from build123d import *

# Parameters (mm, degrees)
BOSS_EXTRUDE1_DEPTH = 5.9944
CUT_EXTRUDE2_DEPTH  = 5.9944


with BuildPart() as part:
    # Sketch1 → Boss-Extrude1 (new body)
    with BuildSketch(Plane.XY):
        Polygon((25.4, 5.9944), (50.8, 5.9944), (50.8, 0), (76.2, 0), (76.2, 5.9944), (101.6, 5.9944), (101.6, 0), (127, 0), (127, 75.4888), (101.6, 75.4888), (101.6, 69.4944), (76.2, 69.4944), (76.2, 75.4888), (50.8, 75.4888), (50.8, 69.4944), (25.4, 69.4944), (25.4, 75.4888), (0, 75.4888), (0, 0), (25.4, 0), align=None)
    extrude(amount=BOSS_EXTRUDE1_DEPTH)

    # Sketch2 → Cut-Extrude2 (cut)
    with BuildSketch(Plane.XY.offset(5.9944)):
        Polygon((36.449, 69.4944), (36.449, 64.4144), (34.163, 64.4144), (34.163, 61.8744), (36.449, 61.8744), (36.449, 58.0644), (39.751, 58.0644), (39.751, 61.8744), (42.037, 61.8744), (42.037, 64.4144), (39.751, 64.4144), (39.751, 69.4944), align=None)
        Polygon((36.449, 5.9944), (39.751, 5.9944), (39.751, 11.0744), (42.037, 11.0744), (42.037, 13.6144), (39.751, 13.6144), (39.751, 17.4244), (36.449, 17.4244), (36.449, 13.6144), (34.163, 13.6144), (34.163, 11.0744), (36.449, 11.0744), align=None)
        Polygon((90.551, 5.9944), (90.551, 11.0744), (92.837, 11.0744), (92.837, 13.6144), (90.551, 13.6144), (90.551, 17.4244), (87.249, 17.4244), (87.249, 13.6144), (84.963, 13.6144), (84.963, 11.0744), (87.249, 11.0744), (87.249, 5.9944), align=None)
        Polygon((90.551, 69.4944), (87.249, 69.4944), (87.249, 64.4144), (84.963, 64.4144), (84.963, 61.8744), (87.249, 61.8744), (87.249, 58.0644), (90.551, 58.0644), (90.551, 61.8744), (92.837, 61.8744), (92.837, 64.4144), (90.551, 64.4144), align=None)
    extrude(amount=-CUT_EXTRUDE2_DEPTH, mode=Mode.SUBTRACT)


solid = part.part
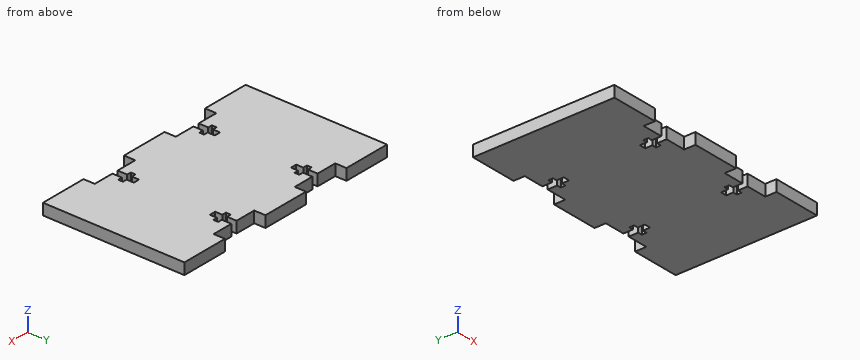
Input: part model. Units: mm. Frame: model coordinates. Coordinates: 2 decimals unless noted, no trailing zeros. Loops run counter-clockwise (first coordinate to the right, second up) from the corner with the lowest first, then second, coordinate; pieces in that order, holes last. Notation, with made-up numbers: (21.25, 50.25) - (67.25, 50.25) arc R31 ccw to (67.25, 80.25) - close; hole circle Ø2 at (1.25, 3.5). An arc over 180 degrees is marked (long way). Answer in a Markdown table with one row per item. Add a question column.
Item 1: Line query: line 1 along X through (y, z) = (70.5, 1.65); line 2 along X through (y, z) = (8.5, 3.8); line 3 along Y through (x, z) = (35.5, 0.8). Output: solid intervals per line, ascending. Write a range as [from, to].
Item 2: Contact query for flat-ended pins moving along their axis: P1, Ø1, axis at x = 15, y = 50, coming from the -Z side; P2, Ø1.1, axis at x = 86, z = 1.5, coming from the -Y side; P3, Ø0.7, axis at x = 91.5, z = 4, coming from the +Y side. Output: stop coordinate, or through.
Item 3: Section query A-A on y = 8. Return the cut outline in (x, z).
Recorded:
| question | item | result |
|---|---|---|
| 1 | line 1 | [0, 25.4], [50.8, 76.2], [101.6, 127] |
| 1 | line 2 | [0, 36.45], [39.75, 87.25], [90.55, 127] |
| 1 | line 3 | [5.99, 11.07], [13.61, 61.87], [64.41, 69.49] |
| 2 | P1 | z = 0 |
| 2 | P2 | y = 5.99 |
| 2 | P3 | y = 69.49 |
| 3 | outline | (0, 0) - (36.45, 0) - (36.45, 5.99) - (0, 5.99) - close; (39.75, 0) - (87.25, 0) - (87.25, 5.99) - (39.75, 5.99) - close; (90.55, 0) - (127, 0) - (127, 5.99) - (90.55, 5.99) - close |
